Input: part model. Units: mm. Frame: model coordinates. Give positions to 0.01 mm unless a question says otherwise; leave off trailing zeros. Order: outer loops, then holes, each group sorted by start corner. A loop starts at its lowest first (then second) coordinate and runs counter-clockwise, first axis right, second up. Notation, with made-up numbers: M 26.25,-24.75 L 51.25,-24.75 A30 ccw 51.25,8.25 Z; hole C 66,-33.5 d4. An arc over 180 degrees is marked long. Use a Markdown table: item, result.
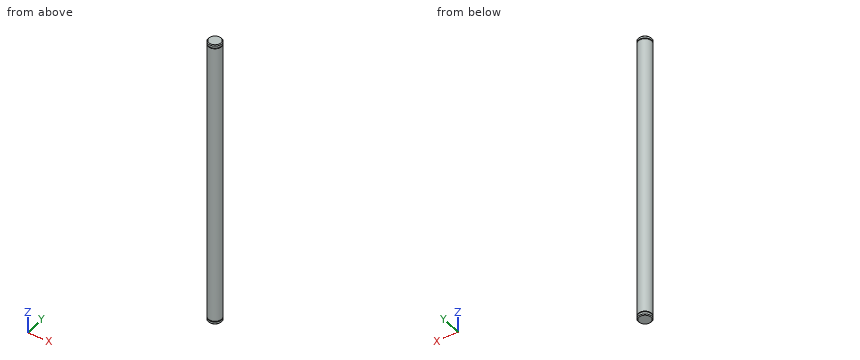
from build123d import *

# Parameters (mm, degrees)
SKETCH1_R                = 6.35
BOSS_EXTRUDE1_DEPTH      = 133.4008
SKETCH2_R                = 5.8547
BOSS_EXTRUDE2_DEPTH      = 0.889
BOSS_EXTRUDE3_START      = 2.54
SKETCH3_R                = 6.35
BOSS_EXTRUDE3_DEPTH      = 2.54
CHAMFER1_SIZE            = 0.762
CHAMFER1_OF_MIRROR1_SIZE = 0.762


with BuildPart() as part:
    # Sketch1 → Boss-Extrude1 (new, symmetric)
    with BuildSketch(Plane.XY):
        Circle(SKETCH1_R)
    extrude(amount=BOSS_EXTRUDE1_DEPTH, both=True)

    # Sketch2 → Boss-Extrude2 (add)
    with BuildSketch(Plane.XY.offset(133.4008)):
        Circle(SKETCH2_R)
    boss_extrude2 = extrude(amount=BOSS_EXTRUDE2_DEPTH)

    # Sketch3 → Boss-Extrude3 (add)
    with BuildSketch(Plane.XY.offset(134.2898).offset(BOSS_EXTRUDE3_START)):
        Circle(SKETCH3_R)
    boss_extrude3 = extrude(amount=-BOSS_EXTRUDE3_DEPTH)

    # Chamfer1
    chamfer1_edges = [part.edges().sort_by_distance(p)[0] for p in [
        (-6.35, 0, 136.8298),
    ]]
    chamfer(chamfer1_edges, length=CHAMFER1_SIZE)

    # Mirror1: Boss-Extrude2, Boss-Extrude3 across plane
    add(boss_extrude2.mirror(Plane.XY))
    add(boss_extrude3.mirror(Plane.XY))

    # Chamfer1 of Mirror1
    chamfer1_of_mirror1_edges = [part.edges().sort_by_distance(p)[0] for p in [
        (-6.35, 0, -136.8298),
    ]]
    chamfer(chamfer1_of_mirror1_edges, length=CHAMFER1_OF_MIRROR1_SIZE)


solid = part.part
1) Cut plane A-A on z = -73.5. Return loops of the section in (x, y).
Response values:
| item | result |
|---|---|
| outline | C 0,0 d12.7 |
2) First-contact query: pin 1 Ø1 at (x, z) = (1, -36.5) entering from +Y; pin 2 Ø2 at (x, z) = (-2.5, -87.5) entering from -Y; pin 3 Ø4 at (y, z) = (2, 20) entering from -X. Flat tips, straight axial feed; report the tip coordinate or a pass-through.
Response values:
| item | result |
|---|---|
| pin 1 | stops at y = 6.33 |
| pin 2 | stops at y = -6.17 |
| pin 3 | stops at x = -6.35 |
3) Material intervals for line 1 (Z direction, x = -5.25, y = 3.5); line 2 (X direction, y = -0.75, z = 113.5); line 3 (Z direction, x = 4.5, y = 4), sorted ascending. Write a range as from..to.
Response values:
| item | result |
|---|---|
| line 1 | z = -136.11..-134.29, -133.4..133.4, 134.29..136.11 |
| line 2 | x = -6.31..6.31 |
| line 3 | z = -136.4..-134.29, -133.4..133.4, 134.29..136.4 |
